```python
from build123d import *

# Parameters (mm, degrees)
PAD_DEPTH       = 3
PAD001_DEPTH    = 3
SKETCH002_W     = 209.08447
SKETCH002_H     = 4.18
PAD002_DEPTH    = 3
SKETCH003_W     = 26.3
SKETCH003_H     = 34.2
POCKET_DEPTH    = 3
SKETCH004_W     = 18
SKETCH004_H     = 25
POCKET001_DEPTH = 3
SKETCH005_W     = 14
SKETCH005_H     = 5
POCKET002_DEPTH = 6


with BuildPart() as part:
    # Sketch → Pad (new body)
    with BuildSketch(Plane.XY):
        with BuildLine():
            ThreePointArc((-100, 50), (-150, 0), (-100, -50))
            Line((-100, -50), (100, -50))
            ThreePointArc((100, -50), (150, 0), (100, 50))
            Line((-100, 50), (100, 50))
        make_face()
    extrude(amount=PAD_DEPTH)

    # Sketch001 (on Face6 of Pad) → Pad001 (join)
    with BuildSketch(Plane.XY.offset(3)):
        with BuildLine():
            ThreePointArc((-100, 50), (-150, 0), (-100, -50))
            Line((-100, -50), (100, -50))
            ThreePointArc((100, -50), (150, 0), (100, 50))
            Line((-100, 50), (100, 50))
        make_face()
        with BuildLine():
            ThreePointArc((-100, 5), (-105, 0), (-100, -5))
            Line((-100, -5), (100, -5))
            ThreePointArc((100, -5), (105, 0), (100, 5))
            Line((-100, 5), (100, 5))
        make_face(mode=Mode.SUBTRACT)
    extrude(amount=PAD001_DEPTH)

    # Sketch002 (on Face9 of Pad001) → Pad002 (join)
    with BuildSketch(Plane.XY.offset(6)):
        with BuildLine():
            ThreePointArc((-100, 50), (-150, 0), (-100, -50))
            Line((-100, -50), (100, -50))
            ThreePointArc((100, -50), (150, 0), (100, 50))
            Line((-100, 50), (100, 50))
        make_face()
        Rectangle(SKETCH002_W, SKETCH002_H, mode=Mode.SUBTRACT)
    extrude(amount=PAD002_DEPTH)

    # Sketch003 (on Face13 of Pad002) → Pocket (cut)
    with BuildSketch(Plane.XY.offset(9)):
        with Locations((0, -29.9)):
            Rectangle(SKETCH003_W, SKETCH003_H)
    extrude(amount=-POCKET_DEPTH, mode=Mode.SUBTRACT)

    # Sketch004 (on Face27 of Pocket) → Pocket001 (cut)
    with BuildSketch(Plane.XY.offset(6)):
        with Locations((0, -25.3)):
            Rectangle(SKETCH004_W, SKETCH004_H)
    extrude(amount=-POCKET001_DEPTH, mode=Mode.SUBTRACT)

    # Sketch005 (on Face13 of Pocket001) → Pocket002 (cut)
    with BuildSketch(Plane.XY.offset(9)):
        with Locations((0, -10.3)):
            Rectangle(SKETCH005_W, SKETCH005_H)
    extrude(amount=-POCKET002_DEPTH, mode=Mode.SUBTRACT)


solid = part.part
```
Design review of the part built by this model. Coordinates are the model's own, in mm. A direction names the side the tool comes from. Coordinates: 2 decimals unless noted, no trailing zeros. Write each loop counter-clockwise with the first axis right and the second up, starting at its lowest first coordinate (ties: lowest second). Pieces come first, ordered by that corner, then holes. Notation, with made-up numbers: M 65.25,-22 L 107.25,-22 A20 cw 107.25,8 Z; hole C 41.5,36 d1. An arc over 180 degrees is marked long. Answer as a JSON object with one key per item and string values.
Item 1: Add section B-B, the plane y = -19. Give the boundary of the cut face in (x, z).
Outcome:
{"outline": "M -146.25,0 L 146.25,0 L 146.25,9 L 13.15,9 L 13.15,6 L 9,6 L 9,3 L -9,3 L -9,6 L -13.15,6 L -13.15,9 L -146.25,9 Z"}
Item 2: Add section A-A, the plane x = 44. Give the boundary of the cut face in (y, z).
Outcome:
{"outline": "M -50,0 L 50,0 L 50,9 L 2.09,9 L 2.09,6 L 5,6 L 5,3 L -5,3 L -5,6 L -2.09,6 L -2.09,9 L -50,9 Z"}
Item 3: Insertion check: pin 1 Ø5 at (y, z) = (21, 3.5) entering from -X; pin 2 Ø0.9 at (y, z) = (-31.5, 7.5) entering from +X; pin 3 Ø3 at (y, z) = (-0.5, 5) entering from -X. Each pin has a flat end and moves straight along its axis. Give the tip position at first contact, or say it passes through.
Outcome:
{"pin 1": "x = -146.45", "pin 2": "x = 139.19", "pin 3": "x = -150"}
Item 4: Wall thickness on probe 1 along Y at (x, z) = (-1, 6.75); probe 2 along Y at (x, z) = (-14, 3.5); probe 3 along Z at (x, y) = (45, 3): over which ranges is each line inside the solid? List them lowest first.
Outcome:
{"probe 1": "-50 to -47, -7.8 to -2.09, 2.09 to 50", "probe 2": "-50 to -5, 5 to 50", "probe 3": "0 to 3, 6 to 9"}
Item 5: Machinability: for faces 4 (the flat face through (-1, -50, 4)), 5 (the cylindrical face through (105, 0, 4)), 6 (the flat face through (-7, -10, 6)), which of the approach directions +Z, -Z, +X, -X, +Y, -Y give a long, thin tool a straight path to every point of the face, cutting with its end or side? Answer none if there is none.
Outcome:
{"face 4": "+Z, -Z, +X, -X, -Y", "face 5": "none", "face 6": "+Z"}
Item 6: Draft analysis for pull direction X (two halves, no side actions). For faces 1 (the flat face through (-1, 50, 4)), 2 (the cylindrical face through (149.988, -1.099, 4.437)), 3 (the flat face through (9, -12.8, 7)), state which applies: pulls with the +X half, pulls with the -X half, needs draft (parallel to the pull), parting line crosses it, or undercut.
Outcome:
{"face 1": "needs draft", "face 2": "pulls with the +X half", "face 3": "undercut"}
Item 7: Add section C-C, the plane z = 1.5. Give the boundary of the cut face in (x, y), and give its area (3 significant figures).
Outcome:
{"outline": "M -100,-50 L 100,-50 A50 ccw 100,50 L -100,50 A50 ccw Z", "area": "27,900 mm²"}
Item 8: Add section D-D, the plane x = 114. Give the boundary of the cut face in (y, z), and give its area (3 significant figures).
Outcome:
{"outline": "M -48,0 L 48,0 L 48,9 L -48,9 Z", "area": "864 mm²"}
